Part model, mm, in its own coordinate system. A direction names the side the tool comes from. Coordinates: 2 decimals unless noted, no trailing zeros. Loops run counter-clockwise (first coordinate to the right, second up) from the corner with the lowest first, then second, coordinate; pieces in that order, holes last. Notation, with made-up numbers: M -11,14.5 L 33,14.5 A22 ccw 33,28.5 Z; hole C 41,0.25 d3. An arc over 180 degrees is marked long. Answer as a JSON object with one key per item and string values. Group by question number.
1. Mould opens along X. For faces 6 (the face through (16.55, -2.81, 84.7)), 7 (the face through (-0.099, -5.972, 30.142)), 8 (the face through (12.425, -1, 15)), 9 (the face through (-0.676, -5.972, 19.536)) say: released by +X, released by -X, zero draft, split by the parting line, or undercut.
2. Saw through at D-D on y = 10.5. Count the separate pieces of the cut face and the enclosed holes in it, then the cut area to 3 significant figures.
3. Drop flat-ended pins along their axis: pin 1 Ø10 at (x, z) = (6.5, 17) entering from +Y; pin 2 Ø4.5 at (x, y) = (8.49, 0.12) entering from +Z; pin 3 Ø12 at (x, y) = (-2, 5.5) entering from -Z; pin 4 Ø6 at (y, z) = (3.5, 32.5) entering from -X. Give the stop position or say it passes through.
4. Saw through at A-A on z = 44.5. Write the cut outline in (x, y) (3 decimals).
5. Saw through at C-C on z = 32.39. Write the cut outline in (x, y) (3 decimals).
6. Saw through at B-B on x = 1. Write the cut outline in (y, z).
7. 3-axis set-ups, long thin cutter, end or side, ignore diameter. For faces 1 (the face through (7.828, 0.883, 65.028)), 2 (the face through (-12.425, -1, 52)), 3 (the face through (-9.559, -0.698, 4.761)), 4 (the face through (12, 6.136, 40)), 5 (the face through (0, 0, 25)): which of +Z, -Z, +X, -X, +Y, -Y reach the whole face in a straight line?
8. Drill centre lines: L1, parallel to Z at x = 0, y = -6.15; L2, parallel to Z at x = 0, y = -1.35; L3, parallel to X at y = -6.15, z = 17.39 (3 decimals). Where is each one in solid material? Low to high.
from build123d import *

# Parameters (mm, degrees)
BOSS_EXTRUDE1_DEPTH           = 75
BOSS_EXTRUDE2_DEPTH           = 25
FILLET1_R                     = 10
CUT_EXTRUDE1_DEPTH            = 117.89311357
CBORE_FOR_M4_SHCS1_AT_2_COUNT = 2
CBORE_FOR_M4_SHCS1_AT_2_PITCH = 15
SKETCH8_R                     = 2
CUT_EXTRUDE2_DEPTH            = 4
SKETCH27_R                    = 2
CUT_EXTRUDE8_DEPTH            = 4
SKETCH29_R                    = 2
CUT_EXTRUDE9_DEPTH            = 2.5
SKETCH30_R                    = 2
CUT_EXTRUDE10_DEPTH           = 2.5
F_6_32_TAPPED_HOLE4_D         = 2.7051
F_6_32_TAPPED_HOLE4_DEPTH     = 9.39
F_6_32_TAPPED_HOLE4_TIP       = 0.81269403
BOSS_EXTRUDE4_DEPTH           = 14.135517109
F_4_40_TAPPED_HOLE1_D         = 2.2606
BOSS_EXTRUDE3_DEPTH           = 60
CUT_EXTRUDE3_DEPTH            = 118.45637488
CUT_EXTRUDE4_DEPTH            = 104.440804328
CUT_EXTRUDE5_DEPTH            = 104.440804328
F_6_32_TAPPED_HOLE3_D         = 2.7051
F_1_72_TAPPED_HOLE1_D         = 1.5113
SKETCH26_W                    = 78.957302066
SKETCH26_H                    = 14.945781294
CUT_EXTRUDE7_DEPTH            = 81.746516953
CUT_EXTRUDE11_START           = 10
SKETCH37_R                    = 4
CUT_EXTRUDE11_DEPTH           = 10


with BuildPart() as part:
    # Sketch1 → Boss-Extrude1 (new body)
    with BuildSketch(Plane.XY):
        Polygon((-3.5, 0), (3.5, 0), (9.425, 6.135517109), (12.425, 6.135517109), (12.425, -8), (-12.425, -8), (-12.425, 6.135517109), (-9.425, 6.135517109), align=None)
    extrude(amount=BOSS_EXTRUDE1_DEPTH)

    # Sketch2 → Boss-Extrude2 (add)
    with BuildSketch(Plane.XY.offset(75)):
        Polygon((-3.5, 0), (-9.425, 6.135517109), (-30, 6.135517109), (-30, -8), (30, -8), (30, 6.135517109), (9.425, 6.135517109), (3.5, 0), align=None)
    extrude(amount=BOSS_EXTRUDE2_DEPTH)

    # Fillet1
    fillet1_edges = [part.edges().sort_by_distance(p)[0] for p in [
        (-12.425, -0.932241445, 75),
        (12.425, -0.932241445, 75),
    ]]
    fillet(fillet1_edges, radius=FILLET1_R)

    # Sketch3 → Cut-Extrude1 (cut, through all)
    with BuildSketch(Plane(origin=(30, 0, 0), x_dir=(0, 0, -1), z_dir=(1, 0, 0))):
        Polygon((-100, -8), (-85.864482891, 6.135517109), (-100, 6.135517109), align=None)
    extrude(amount=-CUT_EXTRUDE1_DEPTH, mode=Mode.SUBTRACT)

    # Sketch6 → CBORE for M4 SHCS1 (revolve, cut)
    with BuildSketch(Plane(origin=(0, 0, 17.39), x_dir=(0, 0, 1), z_dir=(1, 0, 0))):
        Polygon((0, 0), (0, 8), (2.25, 8), (2.25, 4), (4, 4), (4, 0), align=None)
    cbore_for_m4_shcs1 = revolve(axis=Axis((0, 6.35, 17.39), (0, -1, 0)), mode=Mode.SUBTRACT)

    # CBORE for M4 SHCS1 at 2: CBORE for M4 SHCS1 ×2
    with Locations(*[(0, 0, i * CBORE_FOR_M4_SHCS1_AT_2_PITCH) for i in range(1, CBORE_FOR_M4_SHCS1_AT_2_COUNT)]):
        add(cbore_for_m4_shcs1, mode=Mode.SUBTRACT)

    # Sketch8 → Cut-Extrude2 (cut)
    with BuildSketch(Plane(origin=(1.811074119, -1.748933947, 0), x_dir=(0, 0, 1), z_dir=(-0.7193398003386524, 0.6946583704589959, 0))):
        with Locations(Location((5, 6.045178032, 0), (0, 0, 270))):
            Circle(SKETCH8_R)
    extrude(amount=-CUT_EXTRUDE2_DEPTH, mode=Mode.SUBTRACT)

    # Sketch27 → Cut-Extrude8 (cut)
    with BuildSketch(Plane(origin=(-1.811074119, -1.748933947, 0), x_dir=(0, 0, -1), z_dir=(0.7193398003386526, 0.6946583704589958, 0))):
        with Locations(Location((-5, 6.045178032, 0), (0, 0, 90))):
            Circle(SKETCH27_R)
    extrude(amount=-CUT_EXTRUDE8_DEPTH, mode=Mode.SUBTRACT)

    # Sketch29 → Cut-Extrude9 (cut)
    with BuildSketch(Plane(origin=(-1.811074119, -1.748933947, 0), x_dir=(0, 0, -1), z_dir=(0.7193398003386526, 0.6946583704589958, 0))):
        with Locations(Location((-65, 6.045178032, 0), (0, 0, 90))):
            Circle(SKETCH29_R)
    extrude(amount=-CUT_EXTRUDE9_DEPTH, mode=Mode.SUBTRACT)

    # Sketch30 → Cut-Extrude10 (cut)
    with BuildSketch(Plane(origin=(1.811074119, -1.748933947, 0), x_dir=(0, 0, 1), z_dir=(-0.7193398003386524, 0.6946583704589959, 0))):
        with Locations(Location((65, 6.045178032, 0), (0, 0, 270))):
            Circle(SKETCH30_R)
    extrude(amount=-CUT_EXTRUDE10_DEPTH, mode=Mode.SUBTRACT)

    # #6-32 Tapped Hole4
    with Locations(Plane(origin=(0, 0, 0), x_dir=(-1, 0, 0), z_dir=(0, 0, -1))):
        with Locations((-8.485281374, 0.124729477), (8.485281374, 0.124729477)):
            Hole(F_6_32_TAPPED_HOLE4_D / 2, depth=F_6_32_TAPPED_HOLE4_DEPTH)
            with Locations((0, 0, -(F_6_32_TAPPED_HOLE4_DEPTH + F_6_32_TAPPED_HOLE4_TIP / 2))):  # 118° drill point
                Cone(0, F_6_32_TAPPED_HOLE4_D / 2, F_6_32_TAPPED_HOLE4_TIP, mode=Mode.SUBTRACT)

    # Sketch33 → Boss-Extrude4 (add)
    with BuildSketch(Plane(origin=(0, 6.135517109, 0), x_dir=(1, 0, 0), z_dir=(0, 1, 0))):
        with BuildLine():
            Line((-12.425, -30.018095244), (-12.425, -39.981904756))
            ThreePointArc((-12.425, -39.981904756), (-17, -35), (-12.425, -30.018095244))
        make_face()
        with BuildLine():
            Line((12.425, -30.018095244), (12.425, -39.981904756))
            ThreePointArc((12.425, -39.981904756), (17, -35), (12.425, -30.018095244))
        make_face()
    extrude(amount=-BOSS_EXTRUDE4_DEPTH)

    # #4-40 Tapped Hole1 (through all)
    with Locations(Plane(origin=(0, 6.135517109, 0), x_dir=(1, 0, 0), z_dir=(0, 1, 0))):
        with Locations((-12, -35), (12, -35)):
            Hole(F_4_40_TAPPED_HOLE1_D / 2)

    # Sketch9 → Boss-Extrude3 (add)
    with BuildSketch(Plane(origin=(30, 0, 0), x_dir=(0, 0, -1), z_dir=(1, 0, 0))):
        Polygon((-85.864482891, 6.135517109), (-78, 14), (-75, 14), (-75, 6.135517109), align=None)
    extrude(amount=-BOSS_EXTRUDE3_DEPTH)

    # Sketch10 → Cut-Extrude3 (cut, through all)
    with BuildSketch(Plane(origin=(30, 0, 0), x_dir=(0, 0, -1), z_dir=(1, 0, 0))):
        Polygon((-100, -8), (-98, -6), (-98, -8), align=None)
    extrude(amount=-CUT_EXTRUDE3_DEPTH, mode=Mode.SUBTRACT)

    # Sketch11 → Cut-Extrude4 (cut, through all)
    with BuildSketch(Plane(origin=(0, 0, 0), x_dir=(-1, 0, 0), z_dir=(0, 0, -1))):
        Polygon((-3.5, 0), (3.5, 0), (17.019642847, 14), (-17.019642847, 14), align=None)
    extrude(amount=-CUT_EXTRUDE4_DEPTH, mode=Mode.SUBTRACT)

    # Sketch12 → Cut-Extrude5 (cut, through all)
    with BuildSketch(Plane(origin=(0, 0, 0), x_dir=(1, 0, 0), z_dir=(0, 1, 0))):
        with BuildLine():
            Line((3.5, -80), (3.5, -92))
            Line((3.5, -92), (-3.5, -92))
            Line((-3.5, -92), (-3.5, -80))
            ThreePointArc((-3.5, -80), (0, -76.5), (3.5, -80))
        make_face()
    extrude(amount=-CUT_EXTRUDE5_DEPTH, mode=Mode.SUBTRACT)

    # #6-32 Tapped Hole3 (through all)
    with Locations(Plane(origin=(0, 47.060660172, 47.060660172), x_dir=(1, 0, 0), z_dir=(0, 0.7071067811865434, 0.7071067811865517))):
        with Locations((-27, -54.377429751), (27, -54.377429751)):
            Hole(F_6_32_TAPPED_HOLE3_D / 2)

    # #1-72 Tapped Hole1 (through all)
    with Locations(Plane(origin=(0, 47.060660172, 47.060660172), x_dir=(1, 0, 0), z_dir=(0, 0.7071067811865434, 0.7071067811865517))):
        with Locations((-27, -48.877429751), (-27, -59.877429751), (27, -48.877429751), (27, -59.877429751)):
            Hole(F_1_72_TAPPED_HOLE1_D / 2)

    # Sketch26 → Cut-Extrude7 (cut, through all)
    with BuildSketch(Plane(origin=(0, 46, 46), x_dir=(1, 0, 0), z_dir=(0, 0.7071067811865434, 0.7071067811865517))):
        with Locations((0.61611421, -69.350320398)):
            Rectangle(SKETCH26_W, SKETCH26_H)
    extrude(amount=-CUT_EXTRUDE7_DEPTH, mode=Mode.SUBTRACT)

    # Sketch37 → Cut-Extrude11 (cut)
    with BuildSketch(Plane(origin=(0, 0, 0), x_dir=(1, 0, 0), z_dir=(0, 1, 0)).offset(CUT_EXTRUDE11_START)):
        with Locations(Location((0, -17.39, 0), (0, 0, 270))):
            Circle(SKETCH37_R)
        with Locations(Location((0, -32.39, 0), (0, 0, 270))):
            Circle(SKETCH37_R)
    extrude(amount=-CUT_EXTRUDE11_DEPTH, mode=Mode.SUBTRACT)


solid = part.part
Outcome:
{
 "1": {"face 6": "zero draft", "face 7": "undercut", "face 8": "released by +X", "face 9": "undercut"},
 "2": {"separate pieces": "2", "enclosed holes": "2", "area": "208 mm²"},
 "3": {"pin 1": "stops at y = 6.14", "pin 2": "stops at z = 89.75", "pin 3": "stops at z = 0", "pin 4": "stops at x = -17"},
 "4": {"outline": "M -12.425,-8 L 12.425,-8 L 12.425,6.136 L 9.425,6.136 L 3.5,0 L -3.5,0 L -9.425,6.136 L -12.425,6.136 Z"},
 "5": {"outline": "M -16.265,-8 L -2.25,-8 L -2.25,-4 L -4,-4 L -4,0.518 L -9.425,6.136 L -16.265,6.136 Z; M 2.25,-8 L 16.265,-8 L 16.265,6.136 L 9.425,6.136 L 4,0.518 L 4,-4 L 2.25,-4 Z"},
 "6": {"outline": "M -8,0 L 0,0 L 0,13.52 L -4,13.52 L -4,15.37 L -8,15.37 Z; M -8,19.41 L -4,19.41 L -4,21.26 L 0,21.26 L 0,28.52 L -4,28.52 L -4,30.37 L -8,30.37 Z; M -8,34.41 L -4,34.41 L -4,36.26 L 0,36.26 L 0,76.65 L -8,76.65 Z"},
 "7": {"face 1": "none", "face 2": "-X, +Y, -Y", "face 3": "-Z", "face 4": "-Z, +X, -X, +Y", "face 5": "+Z, -Z, +Y"},
 "8": {"L1": "z = 0 to 15.14, 19.64 to 30.14, 34.64 to 76.5", "L2": "z = 0 to 13.39, 21.39 to 28.39, 36.39 to 76.5", "L3": "x = -12.425 to -2.25, 2.25 to 12.425"}
}
